Geometry: see drawing. Coordinates: mm, zero at the bounding-box minimum. A direction names the side the tool comes from. Give positions to 0.01 mm unless a question says otherwise; leave off trailing zeros. Order: outer loops, then holes, each group sorted by start corner. A loop starts at its lowest first (then second) coordinate and runs counter-clockwise, first axis right, second up. Notation, with made-up numbers: M 40.25,-25.5 L 96.25,-25.5 A10 cw 96.25,-21.5 Z; hole C 15.25,41.25 d8. An arc over 180 degrees is marked long. Write item = value, one per line. Start each with the question number.
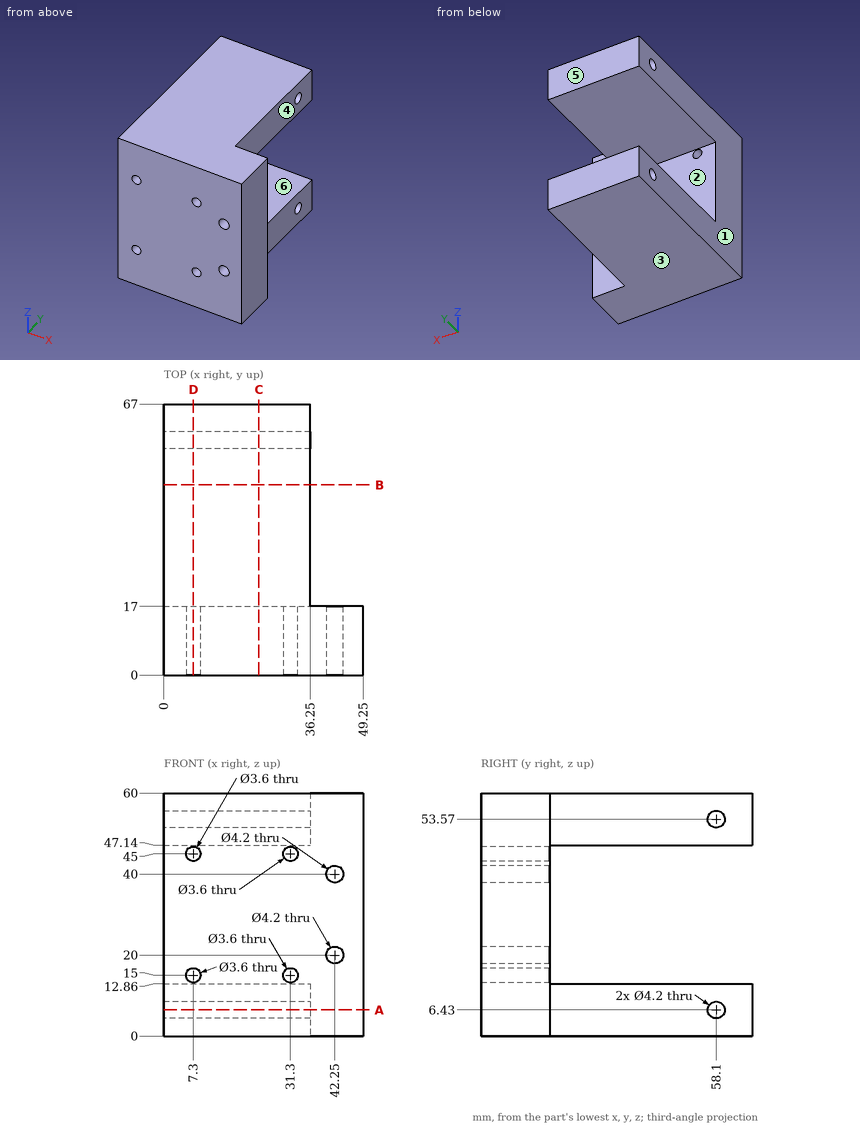
1) Cut plane B-B (y = 47). Return loops of the section in (x, z), plus the area to 3 significant figures.
2) Ray query, L1, parallel to Z at x = 7.3, y = 11.5; L2, parallel to X at y = 7.5, z = 15; L3, parallel to Z at x = 19, y = 19.5. Return the intervals inside material, ascending.
3) Cut plane D-D (x = 7.3). Return loops of the section in (y, z).
4) Draft query along Z for the marked faces 1, 2 and 3. Return one class per face: pulls with the +Z half, pulls with the -Z half, needs draft (parallel to the pull), parting line crosses it, or undercut.
5) Cut plane A-A (z = 6.43). Return loops of the section in (x, y), plus the area to 3 significant figures.
6) Access query for the marked faces 4, 5 and 6. Directions: +Z, -Z, +X, -X, +Y, -Y. A direction counts if a zero-diameter tool reaches every point of the face in a straight line with its end or side. Return the directions, or none.
7) Pin query (flat end, axial travel): pin 1 Ø2 at (x, z) = (7.3, 15) entering from +Y; pin 2 Ø1.5 at (x, z) = (14, 20.5) entering from +Y; pin 3 Ø14 at (y, z) = (49.5, 55.5) entering from +X; pin 4 Ø5 at (x, y) = (36.5, 33) entering from +Z. Return the tip coordinate at first contact, or that it passes through.
8) Cut plane C-C (x = 23.5). Return loops of the section in (y, z), plus the area to 3 significant figures.
Reply:
q1.outline = M 0,0 L 36.25,0 L 36.25,12.86 L 0,12.86 Z; M 0,47.14 L 36.25,47.14 L 36.25,60 L 0,60 Z
q1.area = 932 mm²
q2.L1 = 0 to 13.2, 16.8 to 43.2, 46.8 to 60
q2.L2 = 0 to 5.5, 9.1 to 29.5, 33.1 to 49.25
q2.L3 = 0 to 12.86, 47.14 to 60
q3.outline = M 0,0 L 67,0 L 67,12.86 L 17,12.86 L 17,13.2 L 0,13.2 Z; M 0,16.8 L 17,16.8 L 17,43.2 L 0,43.2 Z; M 0,46.8 L 17,46.8 L 17,47.14 L 67,47.14 L 67,60 L 0,60 Z; hole C 58.1,6.43 d4.2; hole C 58.1,53.57 d4.2
q4.face_1 = needs draft
q4.face_2 = undercut
q4.face_3 = pulls with the -Z half
q5.outline = M 0,0 L 49.25,0 L 49.25,17 L 36.25,17 L 36.25,56 L 0,56 Z; M 0,60.2 L 36.25,60.2 L 36.25,67 L 0,67 Z
q5.area = 2,500 mm²
q6.face_4 = +Z, -Z, +X, +Y
q6.face_5 = +Z, -Z, +X, -X, +Y
q6.face_6 = +X, -X, +Y
q7.pin_1 = through
q7.pin_2 = 17
q7.pin_3 = 36.25
q7.pin_4 = 60
q8.outline = M 0,0 L 67,0 L 67,12.86 L 17,12.86 L 17,47.14 L 67,47.14 L 67,60 L 0,60 Z; hole C 58.1,6.43 d4.2; hole C 58.1,53.57 d4.2
q8.area = 2,280 mm²
